```python
from build123d import *

# Parameters (mm, degrees)
MAINBODY_DEPTH = 304.8


with BuildPart() as part:
    # Sketch2 → MainBody (new body)
    with BuildSketch(Plane.XY):
        with BuildLine():
            Line((-87.11385, -52.07), (87.11385, -52.07))
            Line((87.11385, -52.07), (87.11385, -49.7078))
            Line((87.11385, -49.7078), (85.61385, -49.7078))
            Line((85.61385, -49.7078), (85.61385, -47.3456))
            Line((85.61385, -47.3456), (99.61385, -47.3456))
            Line((99.61385, -47.3456), (99.61385, -49.3141))
            Line((99.61385, -49.3141), (98.11385, -49.3141))
            Line((98.11385, -49.3141), (98.11385, -52.07))
            Line((98.11385, -52.07), (117.82425, -52.07))
            ThreePointArc((117.82425, -52.07), (122.314378061, -50.210128061), (124.17425, -45.72))
            Line((124.17425, -45.72), (124.17425, -41.656))
            Line((124.17425, -41.656), (120.99925, -41.656))
            Line((120.99925, -41.656), (120.99925, -39.6875))
            Line((120.99925, -39.6875), (124.17425, -39.6875))
            Line((124.17425, -39.6875), (124.17425, -35.2171))
            Line((124.17425, -35.2171), (124.968, -35.2171))
            Line((124.968, -35.2171), (124.968, -29.5021))
            Line((124.968, -29.5021), (122.9995, -29.5021))
            Line((122.9995, -29.5021), (122.9995, -31.4706))
            Line((122.9995, -31.4706), (119.0625, -31.4706))
            Line((119.0625, -31.4706), (119.0625, -7.0104))
            Line((119.0625, -7.0104), (122.9995, -7.0104))
            Line((122.9995, -7.0104), (122.9995, -8.9789))
            Line((122.9995, -8.9789), (124.968, -8.9789))
            Line((124.968, -8.9789), (124.968, -3.2639))
            Line((124.968, -3.2639), (124.17425, -3.2639))
            Line((124.17425, -3.2639), (124.17425, 0))
            Line((124.17425, 0), (121.29481323, 0))
            Line((121.29481323, 0), (121.29481323, -4.109997352))
            Line((121.29481323, -4.109997352), (120.011918892, -3.327689915))
            ThreePointArc((120.011918892, -3.327689915), (118.907723578, -2.871189246), (118.671208827, -1.699992881))
            Line((118.671208827, -1.699992881), (114.427, -0.1905))
            Line((114.427, -0.1905), (114.427, -6.5405))
            Line((114.427, -6.5405), (117.475, -6.5405))
            Line((117.475, -6.5405), (117.475, -8.4709))
            Line((117.475, -8.4709), (114.427, -8.4709))
            Line((114.427, -8.4709), (114.427, -10.4013))
            Line((114.427, -10.4013), (117.475, -10.4013))
            Line((117.475, -10.4013), (117.475, -16.3449))
            Line((117.475, -16.3449), (114.427, -16.3449))
            Line((114.427, -16.3449), (114.427, -18.2753))
            Line((114.427, -18.2753), (117.475, -18.2753))
            Line((117.475, -18.2753), (117.475, -20.2057))
            Line((117.475, -20.2057), (114.427, -20.2057))
            Line((114.427, -20.2057), (114.427, -22.1361))
            Line((114.427, -22.1361), (117.475, -22.1361))
            Line((117.475, -22.1361), (117.475, -28.0797))
            Line((117.475, -28.0797), (114.427, -28.0797))
            Line((114.427, -28.0797), (114.427, -30.0101))
            Line((114.427, -30.0101), (117.475, -30.0101))
            Line((117.475, -30.0101), (117.475, -31.9405))
            Line((117.475, -31.9405), (114.427, -31.9405))
            Line((114.427, -31.9405), (114.427, -39.0525))
            ThreePointArc((114.427, -39.0525), (115.382882445, -38.837450889), (115.167833333, -37.881568444))
            Line((115.167833333, -37.881568444), (118.737456339, -36.45102397))
            ThreePointArc((118.737456339, -36.45102397), (121.131104208, -36.728765521), (119.049383871, -37.942491573))
            Line((119.049383871, -37.942491573), (117.82425, -45.72))
            Line((117.82425, -45.72), (121.915072727, -45.72))
            ThreePointArc((121.915072727, -45.72), (120.716898491, -48.612648491), (117.82425, -49.810822727))
            Line((117.82425, -49.810822727), (109.51985, -49.810822727))
            Line((109.51985, -49.810822727), (109.51985, -41.656))
            Line((109.51985, -41.656), (106.21785, -41.656))
            Line((106.21785, -41.656), (106.21785, -43.6118))
            Line((106.21785, -43.6118), (107.15765, -43.6118))
            Line((107.15765, -43.6118), (107.15765, -49.3141))
            Line((107.15765, -49.3141), (101.97605, -49.3141))
            Line((101.97605, -49.3141), (101.97605, -43.6118))
            Line((101.97605, -43.6118), (102.91585, -43.6118))
            Line((102.91585, -43.6118), (102.91585, -41.656))
            Line((102.91585, -41.656), (99.61385, -41.656))
            Line((99.61385, -41.656), (99.61385, -45.0596))
            Line((99.61385, -45.0596), (81.154405407, -45.0596))
            Line((81.154405407, -45.0596), (81.154405407, -49.784))
            Line((81.154405407, -49.784), (-81.154405407, -49.784))
            Line((-81.154405407, -49.784), (-81.154405407, -45.0596))
            Line((-81.154405407, -45.0596), (-99.61385, -45.0596))
            Line((-99.61385, -45.0596), (-99.61385, -41.656))
            Line((-99.61385, -41.656), (-102.91585, -41.656))
            Line((-102.91585, -41.656), (-102.91585, -43.6118))
            Line((-102.91585, -43.6118), (-101.97605, -43.6118))
            Line((-101.97605, -43.6118), (-101.97605, -49.3141))
            Line((-101.97605, -49.3141), (-107.15765, -49.3141))
            Line((-107.15765, -49.3141), (-107.15765, -43.6118))
            Line((-107.15765, -43.6118), (-106.21785, -43.6118))
            Line((-106.21785, -43.6118), (-106.21785, -41.656))
            Line((-106.21785, -41.656), (-109.51985, -41.656))
            Line((-109.51985, -41.656), (-109.51985, -49.810822727))
            Line((-109.51985, -49.810822727), (-117.82425, -49.810822727))
            ThreePointArc((-117.82425, -49.810822727), (-120.716898491, -48.612648491), (-121.915072727, -45.72))
            Line((-121.915072727, -45.72), (-119.049383871, -45.72))
            Line((-119.049383871, -45.72), (-119.049383871, -37.942491573))
            ThreePointArc((-119.049383871, -37.942491573), (-121.131104208, -36.728765521), (-118.737456339, -36.45102397))
            Line((-118.737456339, -36.45102397), (-115.390113559, -38.471235131))
            ThreePointArc((-115.390113559, -38.471235131), (-114.749851886, -38.480556372), (-114.427, -37.927574858))
            Line((-114.427, -37.927574858), (-114.427, -31.9405))
            Line((-114.427, -31.9405), (-117.475, -31.9405))
            Line((-117.475, -31.9405), (-117.475, -30.0101))
            Line((-117.475, -30.0101), (-114.427, -30.0101))
            Line((-114.427, -30.0101), (-114.427, -28.0797))
            Line((-114.427, -28.0797), (-117.475, -28.0797))
            Line((-117.475, -28.0797), (-117.475, -22.1361))
            Line((-117.475, -22.1361), (-114.427, -22.1361))
            Line((-114.427, -22.1361), (-114.427, -20.2057))
            Line((-114.427, -20.2057), (-117.475, -20.2057))
            Line((-117.475, -20.2057), (-117.475, -18.2753))
            Line((-117.475, -18.2753), (-114.427, -18.2753))
            Line((-114.427, -18.2753), (-114.427, -16.3449))
            Line((-114.427, -16.3449), (-117.475, -16.3449))
            Line((-117.475, -16.3449), (-117.475, -10.4013))
            Line((-117.475, -10.4013), (-114.427, -10.4013))
            Line((-114.427, -10.4013), (-114.427, -8.4709))
            Line((-114.427, -8.4709), (-117.475, -8.4709))
            Line((-117.475, -8.4709), (-117.475, -6.5405))
            Line((-117.475, -6.5405), (-114.427, -6.5405))
            Line((-114.427, -6.5405), (-114.427, -0.1905))
            Line((-114.427, -0.1905), (-118.671208827, -1.699992881))
            ThreePointArc((-118.671208827, -1.699992881), (-118.907723578, -2.871189246), (-120.011918892, -3.327689915))
            Line((-120.011918892, -3.327689915), (-121.29481323, -4.109997352))
            Line((-121.29481323, -4.109997352), (-121.29481323, 0))
            Line((-121.29481323, 0), (-124.17425, 0))
            Line((-124.17425, 0), (-124.17425, -3.2639))
            Line((-124.17425, -3.2639), (-124.968, -3.2639))
            Line((-124.968, -3.2639), (-124.968, -8.9789))
            Line((-124.968, -8.9789), (-122.9995, -8.9789))
            Line((-122.9995, -8.9789), (-122.9995, -7.0104))
            Line((-122.9995, -7.0104), (-119.0625, -7.0104))
            Line((-119.0625, -7.0104), (-119.0625, -31.4706))
            Line((-119.0625, -31.4706), (-122.9995, -31.4706))
            Line((-122.9995, -31.4706), (-122.9995, -29.5021))
            Line((-122.9995, -29.5021), (-124.968, -29.5021))
            Line((-124.968, -29.5021), (-124.968, -35.2171))
            Line((-124.968, -35.2171), (-124.17425, -35.2171))
            Line((-124.17425, -35.2171), (-124.17425, -39.6875))
            Line((-124.17425, -39.6875), (-120.99925, -39.6875))
            Line((-120.99925, -39.6875), (-120.99925, -41.656))
            Line((-120.99925, -41.656), (-124.17425, -41.656))
            Line((-124.17425, -41.656), (-124.17425, -45.72))
            ThreePointArc((-124.17425, -45.72), (-122.314378061, -50.210128061), (-117.82425, -52.07))
            Line((-117.82425, -52.07), (-98.11385, -52.07))
            Line((-98.11385, -52.07), (-98.11385, -49.3141))
            Line((-98.11385, -49.3141), (-99.61385, -49.3141))
            Line((-99.61385, -49.3141), (-99.61385, -47.3456))
            Line((-99.61385, -47.3456), (-85.61385, -47.3456))
            Line((-85.61385, -47.3456), (-85.61385, -49.7078))
            Line((-85.61385, -49.7078), (-87.11385, -49.7078))
            Line((-87.11385, -49.7078), (-87.11385, -52.07))
        make_face()
    extrude(amount=MAINBODY_DEPTH)


solid = part.part
```
CAD build for the part. Positions are in the model's coordinates, mm. A direction names the side the tool comes from. Round coordinates to 2 decimals unless told otherwise and drop trailing zeros. Loops run counter-clockwise (first coordinate to the right, second up) from the corner with the lowest first, then second, coordinate; pieces in that order, holes last. Notation, with made-up numbers: M 66.25,-2 L 104.25,-2 A28 cw 104.25,22 Z; hole C 26.25,48 d11. An arc over 180 degrees is marked long. Use a Markdown table: item, result. Add a question column.
(1) Cut at A-A (x = -33). Give the cut face in (y, z), and give its area (3 significant figures).
(2) Which spindle directions (+Z, -Z, +X, -X, +Y, -Y) get a long thin tool onto all of the face, cutting with end or side? Do faces 5 (the face through (91, -45.06, 150)), 6 (the face through (-108, -52.07, 150)), 7 (the face through (-93, -47.346, 150)). Say none if no direction does.
(3) Flat gauge pins, fed straight in: pin 1 (0.6 mm diameter, centred on y = -17.5, z = 138.5, fed in from +X); pin 2 (1.6 mm diameter, centred on y = -42.5, z = 226.5, fed in from -X); pin 3 (1.5 mm diameter, centred on x = -115, z = 217.5, fed in from +Y). Where does each tip first touch, or does it go through?
(4) Drill centre lines: line 1 (X direction, y = -24, z = 283) (1 decimal); line 2 (X direction, y = -22, z = 159); line 3 (X direction, y = -2, z = 133). Where is each one in solid material? Low to high.
(5) Pull direction X, two halves, no side cores. Call faces 1 (the face through (-122.363, -50.16, 150.266)), 2 (the face through (122.265, -50.259, 150.266)), 3 (the face through (114, -49.811, 150)), 4 (the face through (-1, -51, 304.8)): +X half, -X half, draft (parallel to the pull), parting line (faces both ways), or undercut.
Geometry says:
| question | item | result |
|---|---|---|
| 1 | outline | M -52.07,0 L -49.78,0 L -49.78,304.8 L -52.07,304.8 Z |
| 1 | area | 697 mm² |
| 2 | face 5 | +Z, -Z, +Y |
| 2 | face 6 | +Z, -Z, +X, -X, -Y |
| 2 | face 7 | +Z, -Z |
| 3 | pin 1 | stops at x = 119.06 |
| 3 | pin 2 | stops at x = -124.17 |
| 3 | pin 3 | stops at y = -0.19 |
| 4 | line 1 | x = -119.1 to -117.5, 117.5 to 119.1 |
| 4 | line 2 | x = -119.06 to -114.43, 114.43 to 119.06 |
| 4 | line 3 | x = -124.17 to -121.29, -118.62 to -114.43, 114.43 to 118.62, 121.29 to 124.17 |
| 5 | face 1 | -X half |
| 5 | face 2 | +X half |
| 5 | face 3 | undercut |
| 5 | face 4 | draft |
